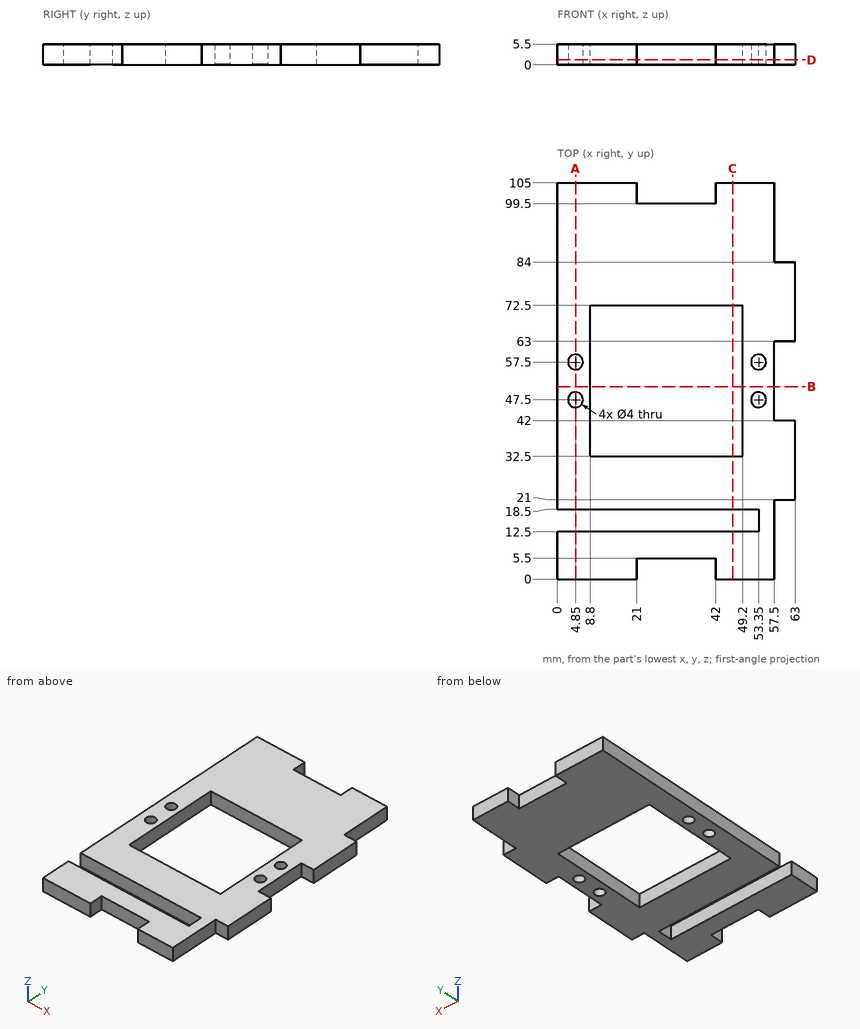
Here's the drawing with two shaded views (mm, measured from the low corner). I have some questions. Round coordinates to 2 decimals unless told otherwise and drop trailing zeros. Loops run counter-clockwise (first coordinate to the right, second up) from the corner with the lowest first, then second, coordinate; pieces in that order, holes last. Notation, with made-up numbers: M 79.25,49.5 L 115.25,49.5 A21 ccw 115.25,80.5 Z; hole C -30.75,-28.5 d8. An arc over 180 degrees is marked long. Answer as a JSON object with one key per item and string values. Group by question number.
Q1. Please list where these lines run through material, in increasing order: L1, parallel to Y at x = 15, z = 1; L2, parallel to Y at x = 40, z = 4.9; L3, parallel to X at y = 59, z = 1.25.
Q2. Will these pins go through, and if not, where does the flat tip stop? pin 1 (1.6 mm diameter, centred on y = 53.5, z = 3, fed in from +X); pin 2 (3 mm diameter, centred on x = 38.5, z = 3.5, fed in from -Y); pin 3 (3 mm diameter, centred on x = 25.5, z = 2, fed in from +Y).
Q3. Imagine slicing it at C-C, the plane x = 46.5. Please give me the cut outline in (y, z).
Q4. Imagine slicing it at A-A, the plane x = 4.85. Please give me the cut outline in (y, z), then the cut area to 4 significant figures.
Q5. Imagine slicing it at B-B, the plane y = 51. Please give me the cut outline in (x, z).
Q6. Imagine slicing it at D-D, the plane z = 1.3. Count the separate pieces of the cut face and the enclosed holes in it, then the cut area to 3 significant figures.
Findings:
{
 "1": {"L1": "y = 0 to 12.5, 18.5 to 32.5, 72.5 to 105", "L2": "y = 5.5 to 12.5, 18.5 to 32.5, 72.5 to 99.5", "L3": "x = 0 to 3.53, 6.17 to 8.8, 49.2 to 52.03, 54.67 to 57.5"},
 "2": {"pin 1": "stops at x = 57.5", "pin 2": "stops at y = 5.5", "pin 3": "stops at y = 99.5"},
 "3": {"outline": "M 0,0 L 12.5,0 L 12.5,5.5 L 0,5.5 Z; M 18.5,0 L 32.5,0 L 32.5,5.5 L 18.5,5.5 Z; M 72.5,0 L 105,0 L 105,5.5 L 72.5,5.5 Z"},
 "4": {"outline": "M 0,0 L 12.5,0 L 12.5,5.5 L 0,5.5 Z; M 18.5,0 L 45.5,0 L 45.5,5.5 L 18.5,5.5 Z; M 49.5,0 L 55.5,0 L 55.5,5.5 L 49.5,5.5 Z; M 59.5,0 L 105,0 L 105,5.5 L 59.5,5.5 Z", "area": "500.5 mm2"},
 "5": {"outline": "M 0,0 L 8.8,0 L 8.8,5.5 L 0,5.5 Z; M 49.2,0 L 57.5,0 L 57.5,5.5 L 49.2,5.5 Z"},
 "6": {"separate pieces": "1", "enclosed holes": "5", "area": "4,050 mm2"}
}
